Source: CAD feature listing. Evaluate the final solid. Frame: model axes, mm. Round coordinates to 2 decimals unless told otherwise and drop trailing zeros. Order: outer loops, then holes, each group sorted by start corner. A loop starts at its lowest first (then second) coordinate and runs counter-clockwise, first axis right, second up. Notation, with made-up numbers: (20, 51) -> (24, 51) arc R14 ccw to (24, 59) -> close; hole circle Ø6 at (47.5, 40.25). An arc over 180 degrees is marked (long way). Answer as CSV lines item,"result". Start each with the question number.
(1) Section query B-B (z = -50.8). Output: boundary loops of the cut face in (x, y) (3 decimals).
(2) Section query D-D (z = 0). Output: boundary loops of the cut face in (x, y) (3 decimals), plus the area to 3 significant figures.
(3) Contact query for flat-ended pins moving along their axis: P1, Ø1, axis at x = 1, z = 38.5, coming from the -Y side; P2, Ø1, axis at x = 1.5, z = -29.5, coming from the +Y side. Output: stop coordinate, or through.
(4) Section query A-A (x = 1.15). Count the separate pieces of the cut face and the enclosed holes in it, plus the area to 3 significant figures.
(5) Section query C-C (y = 25.4). Output: boundary loops of the cut face in (x, z) (3 decimals), plus the area to 3 significant figures.
(6) Line query: line 1 along Y through (x, z) = (1.45, -51) (3 decimals); line 2 along Y through (x, z) = (1.35, 50.8); line 3 along Z through (x, y) = (2.8, 2.5). Output: solid intervals per line, ascending. Write a range as from..to.
```python
from build123d import *

# Parameters (mm, degrees)
SKETCH2_R           = 3.429
SKETCH2_R_2         = 2.54
BOSS_EXTRUDE1_DEPTH = 3.175


with BuildPart() as part:
    # Sketch2 → Boss-Extrude1 (new body)
    with BuildSketch(Plane(origin=(0, 0, 0), x_dir=(0, 0, -1), z_dir=(1, 0, 0))):
        with BuildLine():
            Line((-111.125, 12.7), (18.824359697, 12.7))
            ThreePointArc((18.824359697, 12.7), (20.039379595, 12.941682484), (21.069423728, 13.62993597))
            Line((21.069423728, 13.62993597), (41.434551788, 33.99506403))
            ThreePointArc((41.434551788, 33.99506403), (42.464595921, 34.683317516), (43.679615818, 34.925))
            Line((43.679615818, 34.925), (85.725, 34.925))
            ThreePointArc((85.725, 34.925), (87.97006403, 33.99506403), (88.9, 31.75))
            Line((88.9, 31.75), (88.9, -12.7))
            ThreePointArc((88.9, -12.7), (87.97006403, -14.94506403), (85.725, -15.875))
            Line((85.725, -15.875), (43.679615818, -15.875))
            ThreePointArc((43.679615818, -15.875), (42.464595921, -15.633317516), (41.434551788, -14.94506403))
            Line((41.434551788, -14.94506403), (40.119423728, -13.62993597))
            ThreePointArc((40.119423728, -13.62993597), (39.089379595, -12.941682484), (37.874359697, -12.7))
            Line((37.874359697, -12.7), (-111.125, -12.7))
            ThreePointArc((-111.125, -12.7), (-113.37006403, -11.77006403), (-114.3, -9.525))
            Line((-114.3, -9.525), (-114.3, 9.525))
            ThreePointArc((-114.3, 9.525), (-113.37006403, 11.77006403), (-111.125, 12.7))
        make_face()
        with Locations((-101.6, 0)):
            Circle(SKETCH2_R, mode=Mode.SUBTRACT)
        with Locations((-76.2, 0)):
            Circle(SKETCH2_R, mode=Mode.SUBTRACT)
        with Locations((-50.8, 0)):
            Circle(SKETCH2_R, mode=Mode.SUBTRACT)
        with Locations((-25.4, 0)):
            Circle(SKETCH2_R, mode=Mode.SUBTRACT)
        Circle(SKETCH2_R, mode=Mode.SUBTRACT)
        with Locations((50.8, 25.4)):
            Circle(SKETCH2_R_2, mode=Mode.SUBTRACT)
        with Locations((76.2, 25.4)):
            Circle(SKETCH2_R_2, mode=Mode.SUBTRACT)
        with Locations((50.8, -6.35)):
            Circle(SKETCH2_R_2, mode=Mode.SUBTRACT)
        with Locations((76.2, -6.35)):
            Circle(SKETCH2_R_2, mode=Mode.SUBTRACT)
    extrude(amount=BOSS_EXTRUDE1_DEPTH)


solid = part.part
```
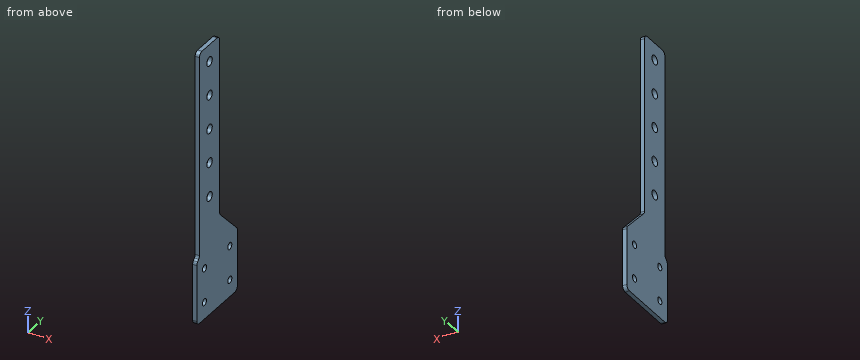
Answer block:
1,outline,"(0, -15.875) -> (3.175, -15.875) -> (3.175, -8.89) -> (0, -8.89) -> close; (0, -3.81) -> (3.175, -3.81) -> (3.175, 22.86) -> (0, 22.86) -> close; (0, 27.94) -> (3.175, 27.94) -> (3.175, 34.925) -> (0, 34.925) -> close"
2,outline,"(0, -12.7) -> (3.175, -12.7) -> (3.175, -3.429) -> (0, -3.429) -> close; (0, 3.429) -> (3.175, 3.429) -> (3.175, 12.7) -> (0, 12.7) -> close"
2,area,"58.9 mm2"
3,P1,"y = -12.7"
3,P2,"y = 22.56"
4,separate pieces,"1"
4,enclosed holes,"9"
4,area,"6,320 mm2"
5,outline,"(0, -88.9) -> (3.175, -88.9) -> (3.175, -78.74) -> (0, -78.74) -> close; (0, -73.66) -> (3.175, -73.66) -> (3.175, -53.34) -> (0, -53.34) -> close; (0, -48.26) -> (3.175, -48.26) -> (3.175, -32.839) -> (0, -32.839) -> close"
5,area,"146 mm2"
6,line 1,"-15.875..-8.882, -3.818..22.868, 27.932..34.925"
6,line 2,"-12.7..-3.43, 3.43..12.7"
6,line 3,"-88.9..-2.35, 2.35..23.05, 27.75..48.45, 53.15..73.85, 78.55..99.25, 103.95..114.3"
